Autodesk Inventor part; units mm, degrees
ref_plane "YZ Plane" through (0, 0, 0) normal (1, 0, 0) x (0, 1, 0)
ref_plane "XZ Plane" through (0, 0, 0) normal (0, 1, 0) x (-1, 0, 0)
ref_plane "Plan de construction4" through (0, 0, 21) normal (0, 0, 1) x (1, 0, 0)
sketch "Esquisse" plane through (0, 0, 21) normal (0, 0, 1) x (1, 0, 0)
  circle A0 centre (0, 0) radius 11.5
  line L0 (16, -11.5) -> (-16, -11.5) construction
  line L1 (-16, -11.5) -> (-16, 38.5)
  line L2 (-16, 38.5) -> (16, 38.5) construction
  line L3 (16, 38.5) -> (16, -11.5)
  line L4 (0, 0) -> (-13.5, 6.75) construction
  circle A1 centre (-13.5, 6.75) radius 1.1 construction
  line L5 (-13.5, 6.75) -> (-13.5, 14.75) construction
  line L6 (-13.5, 14.75) -> (-13.5, 22.75) construction
  line L7 (-13.5, 22.75) -> (-13.5, 30.75) construction
  circle A2 centre (-13.5, 30.75) radius 1.1 construction
  circle A3 centre (-13.5, 22.75) radius 1.1 construction
  circle A4 centre (-13.5, 14.75) radius 1.1 construction
  line L8 (-23.9117, 0) -> (22.6519, 0) construction
  line L9 (10.1, 32.6) -> (10.1, 5.4991) construction
  line L10 (-10.1, 5.4991) -> (-10.1, 32.6) construction
  line L11 (-10.1, 32.6) -> (10.1, 32.6) construction
  line L12 (16, -11.5) -> (0, 0) construction
  line L13 (-16, -11.5) -> (0, 0) construction
  line L14 (10.1, 5.4991) -> (-10.1, 5.4991) construction
  line L15 (16, 38.5) -> (-16, 38.5)
  line L16 (-16, 38.5) -> (-16, 95.5)
  line L17 (-16, 95.5) -> (16, 95.5)
  line L18 (16, 95.5) -> (16, 38.5)
  line L19 (0, -65.3) -> (0, 129.3) construction
  circle A5 centre (13.5, 6.75) radius 1.1 construction
  circle A6 centre (13.5, 30.75) radius 1.1 construction
  circle A7 centre (13.5, 22.75) radius 1.1 construction
  circle A8 centre (13.5, 14.75) radius 1.1 construction
  line L20 (-16, -11.5) -> (16, -11.5) construction
  line L21 (16, -11.5) -> (16, -37.5)
  line L22 (16, -37.5) -> (-16, -37.5)
  line L23 (-16, -37.5) -> (-16, -11.5)
  line L24 (16, 95.5) -> (-16, 95.5)
  line L25 (-16, 95.5) -> (-16, 101.5)
  line L26 (-16, 101.5) -> (16, 101.5)
  line L27 (16, 101.5) -> (16, 95.5)
  line L28 (16, -37.5) -> (-17.2597, -37.5)
  circle A9 centre (-13.5, -6.75) radius 1.1
  circle A10 centre (-13.5, -30.75) radius 1.1
  circle A11 centre (-13.5, -22.75) radius 1.1
  circle A12 centre (-13.5, -14.75) radius 1.1
  line L29 (10.1, -32.6) -> (10.1, -5.4991)
  line L30 (-10.1, -5.4991) -> (-10.1, -32.6)
  line L31 (-10.1, -32.6) -> (10.1, -32.6)
  circle A13 centre (13.5, -6.75) radius 1.1
  circle A14 centre (13.5, -14.75) radius 1.1
  circle A15 centre (13.5, -22.75) radius 1.1
  circle A16 centre (13.5, -30.75) radius 1.1
  line L32 (10.1, -32.6) -> (10.1, -5.4991)
  line L33 (-10.1, -5.4991) -> (-10.1, -32.6)
  line L34 (-10.1, -32.6) -> (10.1, -32.6)
  circle A17 centre (0, 50) radius 1.55
  circle A18 centre (-13.5, 56.75) radius 1.1
  circle A19 centre (-13.5, 64.75) radius 1.1
  circle A20 centre (-13.5, 72.75) radius 1.1
  circle A21 centre (-13.5, 80.75) radius 1.1
  circle A22 centre (13.5, 56.75) radius 1.1
  circle A23 centre (13.5, 64.75) radius 1.1
  circle A24 centre (13.5, 80.75) radius 1.1
  circle A25 centre (13.5, 72.75) radius 1.1
  line L35 (-13.5, 56.75) -> (-13.5, 64.75) construction
  line L36 (-13.5, 72.75) -> (-13.5, 64.75) construction
  line L37 (-13.5, 80.75) -> (-13.5, 72.75) construction
  line L38 (-13.5, 30.75) -> (-13.5, 56.75) construction
  line L39 (13.5, 56.75) -> (13.5, 64.75) construction
  line L40 (13.5, 64.75) -> (13.5, 72.75) construction
  line L41 (13.5, 72.75) -> (13.5, 80.75) construction
  line L42 (-13.5, 80.75) -> (13.5, 80.75) construction
  line L43 (-9, 69) -> (9, 69)
  line L44 (9, 69) -> (9, 60)
  line L45 (9, 60) -> (-9, 60)
  line L46 (-9, 60) -> (-9, 69)
  line L47 (-9, 69) -> (9, 60) construction
  line L48 (9, 69) -> (-9, 60) construction
  line L49 (16, 54.75) -> (11.5, 54.75)
  line L50 (11.5, 54.75) -> (11.5, 83.85)
  line L51 (11.5, 83.85) -> (-11.5, 83.85)
  line L52 (-11.5, 83.85) -> (-11.5, 54.75)
  line L53 (-11.5, 54.75) -> (-16, 54.75)
  line L54 (16, 85.85) -> (-16, 85.85)
  line L55 (0, 50) -> (-11, 50) construction
  line L56 (-11, 50) -> (-11, 39) construction
  circle A26 centre (-11, 50) radius 1.55
  circle A27 centre (-11, 39) radius 1.55
  point P0 (0, -11.5)
  point P1 (16, -11.5)
  point P2 (10.1, -5.4991)
  point P3 (0, 64.5)
  dimension "d107" = 23
  dimension "d133" = 6.75
  dimension "d135" = 2.2
  dimension "d137" = 8
  dimension "d138" = 20.2
  dimension "d160" = 50
  dimension "d161" = 5.9
  dimension "d162" = 32
  dimension "d163" = 11.5
  dimension "d169" = 26
  dimension "d224" = 57
  dimension "d225" = 6
  dimension "d240" = 13.5
  dimension "d247" = 95.5
  dimension "d248" = 133
  dimension "d249" = 50
  dimension "d250" = 3.1
  dimension "d254" = 6.75
  dimension "d255" = 8
  dimension "d256" = 2.2
  dimension "d257" = 6.75
  dimension "d258" = 10
  dimension "d259" = 9
  dimension "d260" = 18
  dimension "d261" = 2
  dimension "d262" = 2
  dimension "d263" = 2
  dimension "d264" = 2
  dimension "d267" = 3.1
  dimension "d268" = 11
  dimension "d269" = 11
extrude "Face fixation moteur" add sketch "Esquisse" against normal blind 4 contours L1 L15 A27 L3 L21 L22 L23 | L16 L53 L52 L51 L50 L49 L18 L15 A27 | L16 L54 L18 L49 L50 L51 L52 L53 | L16 L17 L18 L54
extrude "Creux moteur" [suppressed]
extrude "Rai basl" add sketch "Esquisse" against normal blind 45 contours L25 L26 L27 L17
sketch "Esquisse16" plane through (-16, 95.5, 17) normal (0, -1, 0) x (1, 0, 0)
  line L0 (0, 0) -> (0, -41)
  line L1 (32, -41) -> (0, -41)
  line L2 (32, 0) -> (32, -41)
  line L3 (5, -6) -> (27, -6) construction
  line L4 (27, -6) -> (27, -31) construction
  line L5 (27, -31) -> (5, -31) construction
  line L6 (5, -31) -> (5, -6) construction
  line L7 (0, 0) -> (0, -41)
  line L8 (0, -1) -> (5, -6) construction
  line L9 (5, -31) -> (0, -36) construction
  line L10 (0, -41) -> (32, -41)
  line L11 (27, -31) -> (32, -36) construction
  circle A0 centre (5, -6) radius 2.1
  circle A1 centre (27, -6) radius 2.1
  circle A2 centre (27, -31) radius 2.1
  circle A3 centre (5, -31) radius 2.1
  line L12 (6.1207, -10.1826) -> (1.9381, -9.0619)
  line L13 (1.9381, -9.0619) -> (0.8174, -4.8793)
  line L14 (0.8174, -4.8793) -> (3.8793, -1.8174)
  line L15 (3.8793, -1.8174) -> (8.0619, -2.9381)
  line L16 (8.0619, -2.9381) -> (9.1826, -7.1207)
  line L17 (9.1826, -7.1207) -> (6.1207, -10.1826)
  line L18 (9.1826, -29.8793) -> (8.0619, -34.0619)
  line L19 (8.0619, -34.0619) -> (3.8793, -35.1826)
  line L20 (3.8793, -35.1826) -> (0.8174, -32.1207)
  line L21 (0.8174, -32.1207) -> (1.9381, -27.9381)
  line L22 (1.9381, -27.9381) -> (6.1207, -26.8174)
  line L23 (6.1207, -26.8174) -> (9.1826, -29.8793)
  line L24 (25.8793, -26.8174) -> (30.0619, -27.9381)
  line L25 (30.0619, -27.9381) -> (31.1826, -32.1207)
  line L26 (31.1826, -32.1207) -> (28.1207, -35.1826)
  line L27 (28.1207, -35.1826) -> (23.9381, -34.0619)
  line L28 (23.9381, -34.0619) -> (22.8174, -29.8793)
  line L29 (22.8174, -29.8793) -> (25.8793, -26.8174)
  line L30 (22.8174, -7.1207) -> (23.9381, -2.9381)
  line L31 (23.9381, -2.9381) -> (28.1207, -1.8174)
  line L32 (28.1207, -1.8174) -> (31.1826, -4.8793)
  line L33 (31.1826, -4.8793) -> (30.0619, -9.0619)
  line L34 (30.0619, -9.0619) -> (25.8793, -10.1826)
  line L35 (25.8793, -10.1826) -> (22.8174, -7.1207)
  line L36 (7.6517, -8.6517) -> (24.3483, -8.6517) construction
  line L37 (24.3483, -8.6517) -> (24.3483, -28.3483) construction
  line L38 (24.3483, -28.3483) -> (7.6517, -28.3483) construction
  line L39 (7.6517, -28.3483) -> (7.6517, -8.6517) construction
  line L40 (32, 4) -> (0, 4)
  line L41 (32, 0) -> (32, -41)
  line L42 (0, 0) -> (0, -41)
  line L43 (0, 4) -> (32, 4)
  line L44 (0, -1) -> (32, -1)
  line L45 (32, -1) -> (27, -6) construction
  line L46 (0, 0) -> (32, 0)
  line L47 (32, -36) -> (0, -36)
  point P0 (16, -17)
  point P1 (28.4, 4)
  point P2 (30.6, 4)
  point P3 (28.4, 4)
  point P4 (30.6, 4)
  point P5 (1.4, 4)
  point P6 (3.6, 4)
  point P7 (1.4, 4)
  point P8 (3.6, 4)
  point P9 (1.4, 4)
  point P10 (3.6, 4)
  point P11 (1.4, 4)
  point P12 (3.6, 4)
  point P13 (28.4, 4)
  point P14 (30.6, 4)
  point P15 (28.4, 4)
  point P16 (30.6, 4)
  dimension "d228" = 5
  dimension "d230" = 4.2
  dimension "d231" = 7.5
  dimension "d232" = 25
  dimension "d233" = 22
  dimension "d245" = 45
  dimension "d246" = 32
  dimension "d251" = 1
  dimension "d253" = 5
extrude "Extrusion23" cut sketch "Esquisse16" against normal through all contours A0 | A1 | A2 | A3
extrude "Extrusion25" add sketch "Esquisse" against normal blind 8.5 contours L16 L54 L18 L49 L50 L51 L52 L53
properties part number "Support AX 12A haut"
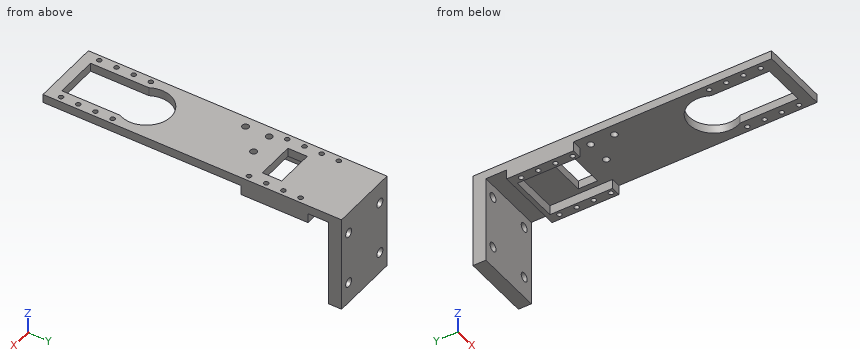
Geometry check sheet. Reference: the model listing, model coordinates, mm. Give positions to 0.01 mm unless a question says otherwise; leave off trailing zeros. Loops run counter-clockwise (first coordinate to the right, second up) from the corner with the lowest first, then second, coordinate; pieces in that order, holes last. Notation, with made-up numbers: M 33.25,21.25 L 78.25,21.25 A27 ccw 78.25,39.25 Z; hole C 63,68.5 d9. An arc over 180 degrees is marked long. Write item = value, one per line. Start each with the question number.
1. Section check A-A, the plane z = 15. Give the number of separate pieces and of enclosed holes in the cut face, plus the area to 3 significant figures.
2. Section check B-B, the plane y = 39. Enter the section's corners in (x, z).
3. Thickness scan on probe 1 along Y at (x, z) = (0, 19); probe 2 along Z at (x, y) = (-11, 97); probe 3 along X at (y, z) = (72.75, 18). Record the ranges inside material, lowest first.
4. Section check C-C, the plane y = -20. Enter the section's corners in (x, z).
5. Go/stop test with flat-tipped pins: P1, Ø5, axis at x = -11, z = -14, coming from the -Y side; P2, Ø2, axis at x = 13.5, y = 80.75, coming from the +Z side; P3, Ø9.5, axis at x = 6.5, y = 75.5, coming from the -Z side; P4, Ø3.5, axis at x = 13.5, y = 72.75, coming from the -Z side. Record where each tip stops, or that it passes through.
6. Section check D-D, the plane z = -9.5. Enter the section's corners in (x, y), plus the area to 3 significant figures.
Values follow:
q1.separate_pieces = 2
q1.enclosed_holes = 8
q1.area = 487 mm^2
q2.outline = M -16,17 L -12.55,17 L -12.55,21 L -16,21 Z; M -9.45,17 L 16,17 L 16,21 L -9.45,21 Z
q3.probe_1 = -37.5 to -32.6, 11.5 to 48.45, 51.55 to 60, 69 to 101.5
q3.probe_2 = -24 to -16.1, -11.9 to 8.9, 13.1 to 21
q3.probe_3 = -16 to -14.6, -12.4 to 12.4, 14.6 to 16
q4.outline = M -16,17 L -10.1,17 L -10.1,21 L -16,21 Z; M 10.1,17 L 16,17 L 16,21 L 10.1,21 Z
q5.P1 = 95.5
q5.P2 = through
q5.P3 = 17
q5.P4 = 12.5
q6.outline = M -16,95.5 L 16,95.5 L 16,101.5 L -16,101.5 Z
q6.area = 192 mm^2
